Geometry: final body of the model. Coordinates: model frame, mm. Face numbers are marked on the shaded views. A direction names the side the tool comes from. Give positions to 0.01 mm unless a question says otherwise; leave off trailing zeros. Loops run counter-clockwise (first coordinate to the right, second up) from the corner with the lowest first, then second, coordinate; pieces in that order, holes last.
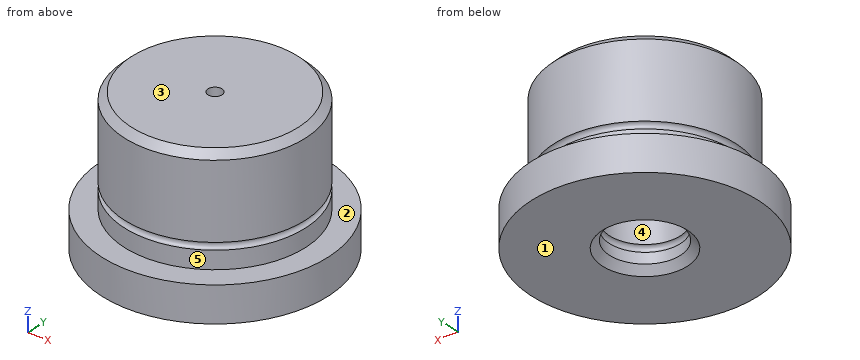
from build123d import *

# Parameters (mm, degrees)
F2_SIZE = 1
F3_SIZE = 1


with BuildPart() as f1:
    # F0 (on Front) → F1 (revolve)
    with BuildSketch(Plane.XZ):
        with BuildLine():
            Line((12.8, 0), (1, 0))
            Line((1, 0), (1, -5))
            Line((1, -5), (5, -10))
            Line((5, -10), (5, -16.5))
            ThreePointArc((5, -16.5), (5.5, -17), (5, -17.5))
            Line((5, -17.5), (5, -20))
            Line((5, -20), (16, -20))
            Line((16, -20), (16, -15))
            Line((16, -15), (12.8, -15))
            Line((12.8, -15), (12.8, -12.5))
            ThreePointArc((12.8, -12.5), (12.3, -12), (12.8, -11.5))
            Line((12.8, -11.5), (12.8, 0))
        make_face()
    revolve(axis=Axis((0, 0, -16.444752), (0, 0, -1)))

    # F2
    f2_edges = [f1.edges().sort_by_distance(p)[0] for p in [
        (-12.8, 0, 0),
    ]]
    chamfer(f2_edges, length=F2_SIZE)

    # F3
    f3_edges = [f1.edges().sort_by_distance(p)[0] for p in [
        (-5, 0, -20),
    ]]
    chamfer(f3_edges, length=F3_SIZE)


solid = f1.part
Item 1: Pin query (flat end, axial travel): pin 1 (10 mm diameter, centred on x = -7, z = -16, fed in from +Y); pin 2 (12 mm diameter, centred on x = -6.5, z = -7.5, fed in from +Y); pin 3 (1.5 mm diameter, centred on x = -8, z = -3.5, fed in from +Y); pin 4 (1.6 mm diameter, centred on x = 0, y = 0, fed in from +Z). Return the tip coordinate at first contact, or that it passes through.
Values follow:
pin 1: stops at y = 15.87
pin 2: stops at y = 12.79
pin 3: stops at y = 10.55
pin 4: passes through
Item 2: Section query A-A on y = 0. Return loops of the section in (x, z).
Values follow:
outline: (-16, -20) - (-6, -20) - (-5, -19) - (-5, -17.5) arc R0.5 cw to (-5, -16.5) - (-5, -10) - (-1, -5) - (-1, 0) - (-11.8, 0) - (-12.8, -1) - (-12.8, -11.5) arc R0.5 cw to (-12.8, -12.5) - (-12.8, -15) - (-16, -15) - close; (1, -5) - (5, -10) - (5, -16.5) arc R0.5 cw to (5, -17.5) - (5, -19) - (6, -20) - (16, -20) - (16, -15) - (12.8, -15) - (12.8, -12.5) arc R0.5 cw to (12.8, -11.5) - (12.8, -1) - (11.8, 0) - (1, 0) - close
Item 3: Section query D-D on z = -18.5. Return loops of the section in (x, y), plus the area to 3 significant figures.
Values follow:
outline: circle Ø32 at (0, 0); hole circle Ø10 at (0, 0)
area: 726 mm2
Item 4: Ray query, probe 1 along Y at (x, z) = (0, -3); probe 2 along Y at (x, z) = (0, -13.5). Return the intervals inside material, ascending.
Values follow:
probe 1: y = -12.8 to -1, 1 to 12.8
probe 2: y = -12.8 to -5, 5 to 12.8
Item 5: Draft query along X for the marked faces 3, 4 and 5. Return one class per face: +X half, -X half, draft (parallel to the pull), parting line (faces both ways), or undercut.
Values follow:
face 3: draft
face 4: undercut
face 5: parting line
Item 6: Section query C-C on z = -4.5. Return loops of the section in (x, y), plus the area to 3 significant figures.
Values follow:
outline: circle Ø25.6 at (0, 0); hole circle Ø2 at (0, 0)
area: 512 mm2
Item 7: Set-up query: the marked faces 1 and 2. Return all of +Z, -Z, +X, -X, +Y, -Y with unobstructed straight access to the full face (end or side cutting, diameter ignored); none if empty.
Values follow:
face 1: -Z, +X, -X, +Y, -Y
face 2: +Z
